Solid Edge part; units mm, degrees
sketch "Sketch1" plane through (0, 0, 0) normal (0, 0, 1) x (1, 0, 0)
  line L0 (-1, -40) -> (1, -40)
  line L1 (1, -40) -> (1, 40)
  line L2 (1, 40) -> (-1, 40)
  line L3 (-1, 40) -> (-1, -40)
  dimension "D1" = 1
  dimension "D2" = 1
extrude "Protrusion1" add sketch "Sketch1" along normal blind 24.8
sketch "Sketch2" plane through (0, -40, 8) normal (0, -1, 0) x (0, 0, 1)
  line L0 (-8, -1) -> (-8, -16)
  line L1 (-8, -16) -> (4.4, -8.8409)
  line L2 (4.4, -8.8409) -> (16.8, -16)
  line L3 (16.8, -16) -> (16.8, -1)
  dimension "D1" = 16.8
extrude "Protrusion2" add sketch "Sketch2" against normal up to vertex (80 mm away) material side at (8.5, -40, 0.05)
sketch "Sketch3" plane through (-1, 0, 12.4) normal (-1, 0, 0) x (0, 0, 1)
  circle A0 centre (-5, 27.5) radius 1.875
  circle A1 centre (-5, -27.5) radius 1.875
  dimension "D1" = 5
extrude "Extrusionsausschnitt_5" cut sketch "Sketch3" against normal blind 8
sketch "Sketch4" plane through (7.5, 40, 12.4) normal (0, 1, 0) x (0, 0, 1)
  line L0 (-12.4, 6.3409) -> (12.4, 6.3409)
extrude "Cutout1" cut sketch "Sketch4" against normal through all material side at (13.8909, 40, 12.4)
chamfer "Fase_1" distance 0.3 angle 45 2 edges at (-1, 27.5, 5.525) (-1, -27.5, 5.525)
properties material "Polypropylen, allgemein"
Input: part model. Units: mm. Frame: model coordinates. A direction names the side the tool comes from. Coordinates: 2 decimals unless noted, no trailing zeros. Loops run counter-clockwise (first coordinate to the right, second up) from the corner with the lowest first, then second, coordinate; pieces in that order, holes last.
(1) First-contact query: pin 1 Ø1.9 at (y, z) = (28, 7) entering from -X; pin 2 Ø6 at (y, z) = (-27.5, 7.4) entering from +X; pin 3 Ø4.5 at (y, z) = (27.5, 7.4) entering from +X. Flat tips, straight axial feed; report the tip coordinate or a pass-through.
(2) Material intervals for probe 1 along Y at (x, z) = (1.25, 7.4) (3 decimals); probe 2 along Y at (x, z) = (6, 8.5); probe 3 along Z at (x, y) = (10.75, 21), sorted ascending.
(3) Section A-A on y = 27.5. Return the cut outline in (x, z) (3 decimals), then the cut area to 3 significant figures.
(4) Section C-C on y = -1. Return the cut outline in (x, z), then the cut area to 3 significant figures.
(5) Section B-B on z = 7.4. Return the cut outline in (x, y) (3 decimals), then the cut area to 3 significant figures.
(6) Section D-D on z = 13.25. Return the cut outline in (x, y).
(7) Pull-direction query (Z, two-part tool) for faces 4 (the face through (6, 1, 24.8)), 5 (the face through (11.306, -0.56, 16.67)), 6 (the face through (6, 1, 0)), 7 (the face through (7, 40, 12)); classes: released by +Z, released by -Z, zero draft, split by the parting line, or undercut.
(8) Set-up query: faces 1 (the face through (11.376, -0.56, 8.009)), 2 (the face through (7, 27, 7)), 3 (the face through (-1, 1, 12)). Return all of +Z, -Z, +X, -X, +Y, -Y with unobstructed straight access to the full face (end or side cutting, diameter ignored); none if empty.
Data:
1. pin 1: stops at x = 7
1. pin 2: stops at x = 13.46
1. pin 3: stops at x = 13.03
2. probe 1: y = -40 to -29.375, -25.625 to 25.625, 29.375 to 40
2. probe 2: y = -40 to -29.02, -25.98 to 25.98, 29.02 to 40
2. probe 3: z = 0 to 9.09, 15.71 to 24.8
3. outline: (-1, 0) - (13.841, 0) - (13.841, 3.74) - (8.841, 12.4) - (13.841, 21.06) - (13.841, 24.8) - (-1, 24.8) - (-1, 9.575) - (-0.7, 9.275) - (7, 9.275) - (7, 5.525) - (-0.7, 5.525) - (-1, 5.225) - close
3. area: 295 mm2
4. outline: (-1, 0) - (13.84, 0) - (13.84, 3.74) - (8.84, 12.4) - (13.84, 21.06) - (13.84, 24.8) - (-1, 24.8) - close
4. area: 325 mm2
5. outline: (-1, -40) - (11.728, -40) - (11.728, 40) - (-1, 40) - (-1, 29.675) - (-0.7, 29.375) - (7, 29.375) - (7, 25.625) - (-0.7, 25.625) - (-1, 25.325) - (-1, -25.325) - (-0.7, -25.625) - (7, -25.625) - (7, -29.375) - (-0.7, -29.375) - (-1, -29.675) - close
5. area: 958 mm2
6. outline: (-1, -40) - (9.33, -40) - (9.33, 40) - (-1, 40) - close
7. face 4: released by +Z
7. face 5: undercut
7. face 6: released by -Z
7. face 7: zero draft
8. face 1: +X, +Y, -Y
8. face 2: -X
8. face 3: +Z, -Z, -X, +Y, -Y
